CAD build for the part. Positions are in the model's coordinates, mm. A direction names the side the tool comes from. Round coordinates to 2 decimals unless told otherwise and drop trailing zeros. Write each loop counter-clockwise with the first axis right and the second up, starting at its lowest first coordinate (ties: lowest second). Pieces come first, ordered by that corner, then holes. Notation, with made-up numbers: (36, 57.25) - (73, 57.25) arc R8 cw to (73, 71.25) - close; hole circle Ø5 at (20, 67). An arc over 180 degrees is marked (long way). Put each result on its own line as item: value. Start each with the question number.
Item 1: Mould opens along X. For faces 5 (the flat face through (50.364, 6, 0)), 6 (the flat face through (16, -3, -4.645)), 7 (the cylindrical face through (55.35, 0.74, -8.24)) say: released by +X, released by -X, zero draft, split by the parting line, or undercut.
Item 2: Cut at C-C (z = -1). Give the cut face in (x, y), and give its area (3 significant figures).
Item 3: Pin check, flat tips, straight feed: pin 1 Ø3 at (x, z) = (-0.5, 4) entering from +Y; pin 2 Ø5.5 at (y, z) = (-4.5, 6.5) entering from -X; pin 3 Ø4 at (y, z) = (-3, -1.5) entering from +X. Stop position of each tip, or through.
Item 4: Cut at B-B (x = -14). Give the cut face in (y, z).
Item 5: Drill centre lines: line 1 (Y direction, x = -9.5, z = -4.5); line 2 (Y direction, x = -14, z = 6); line 3 (X direction, y = -0.5, z = -4). Where is each one in solid material? Low to high. Write a range as from..to.
Item 6: Cut at A-A (z = 18.5). Give the cut face in (x, y).
Item 7: 3-axis set-ups, long thin cutter, end or side, ignore diameter. For faces 1 (the flat face through (8.364, 6, 0)), 2 (the flat face through (51.864, -3, 7)), 3 (the flat face through (29, 6, 9.755)), 4 (the flat face through (16, -6.9, 8)): which of +Z, -Z, +X, -X, +Y, -Y reach the whole face in a straight line?
Item 8: Cut at D-D (y = -3.5). Give the cut face in (x, z).
```python
from build123d import *

# Parameters (mm, degrees)
SKETCH_1_W          = 80
SKETCH_1_H          = 36
SKETCH_1_R          = 1.5
EXTRUDE_1_DEPTH     = 1.5
SKETCH_2_W          = 71
SKETCH_2_H          = 24.2
EXTRUDE_2_DEPTH     = 7
SKETCH_3_W          = 42
SKETCH_3_H          = 19.2
EXTRUDE_3_DEPTH     = 9
SKETCH_4_W          = 64.4
SKETCH_4_H          = 14.5
CUT_EXTRUDE_1_DEPTH = 0.1


with BuildPart() as part:
    # Эскиз1 → Бобышка-Вытянуть1 (new body)
    with BuildSketch(Plane(origin=(0, 0, 0), x_dir=(1, 0, 0), z_dir=(0, 1, 0))):
        with Locations((16.363636364, -7.454545455)):
            Rectangle(SKETCH_1_W, SKETCH_1_H)
        with Locations(Location((-21.136363636, -22.954545455, 0), (0, 0, 270))):
            Circle(SKETCH_1_R, mode=Mode.SUBTRACT)
        with Locations(Location((53.863636364, 8.045454545, 0), (0, 0, 270))):
            Circle(SKETCH_1_R, mode=Mode.SUBTRACT)
        with Locations(Location((-21.136363636, 8.045454545, 0), (0, 0, 270))):
            Circle(SKETCH_1_R, mode=Mode.SUBTRACT)
        with Locations(Location((53.863636364, -22.954545455, 0), (0, 0, 270))):
            Circle(SKETCH_1_R, mode=Mode.SUBTRACT)
    extrude(amount=EXTRUDE_1_DEPTH)

    # Эскиз2 → Бобышка-Вытянуть2 (add)
    with BuildSketch(Plane.XZ):
        with Locations((16.363636364, 7.454545455)):
            Rectangle(SKETCH_2_W, SKETCH_2_H)
    extrude(amount=EXTRUDE_2_DEPTH)

    # Эскиз3 → Бобышка-Вытянуть3 (add)
    with BuildSketch(Plane(origin=(0, 1.5, 0), x_dir=(1, 0, 0), z_dir=(0, 1, 0))):
        with Locations((29.363636364, -0.154545455)):
            Rectangle(SKETCH_3_W, SKETCH_3_H)
    extrude(amount=EXTRUDE_3_DEPTH)

    # Эскиз4 → Вырез-Вытянуть1 (cut)
    with BuildSketch(Plane.XZ.offset(7)):
        with Locations((16.363636364, 7.454545455)):
            Rectangle(SKETCH_4_W, SKETCH_4_H)
    extrude(amount=-CUT_EXTRUDE_1_DEPTH, mode=Mode.SUBTRACT)


solid = part.part
```
Output values:
1. face 5: released by +X
1. face 6: zero draft
1. face 7: undercut
2. outline: (-23.64, 0) - (-19.14, 0) - (-19.14, -7) - (51.86, -7) - (51.86, 0) - (56.36, 0) - (56.36, 1.5) - (50.36, 1.5) - (50.36, 10.5) - (8.36, 10.5) - (8.36, 1.5) - (-23.64, 1.5) - close
2. area: 995 mm2
3. pin 1: y = 1.5
3. pin 2: x = -19.14
3. pin 3: x = 51.86
4. outline: (-7, -4.65) - (0, -4.65) - (0, -10.55) - (1.5, -10.55) - (1.5, 25.45) - (0, 25.45) - (0, 19.55) - (-7, 19.55) - (-7, 14.7) - (-6.9, 14.7) - (-6.9, 0.2) - (-7, 0.2) - close
5. line 1: -7..1.5
5. line 2: -6.9..1.5
5. line 3: -19.14..51.86
6. outline: (-23.64, 0) - (-19.14, 0) - (-19.14, -7) - (51.86, -7) - (51.86, 0) - (56.36, 0) - (56.36, 1.5) - (-23.64, 1.5) - close
7. face 1: +Z, -Z, -X, +Y
7. face 2: +Z, -Z, +X, -Y
7. face 3: +Z, +X, -X, +Y
7. face 4: -Y
8. outline: (-19.14, -4.65) - (51.86, -4.65) - (51.86, 19.55) - (-19.14, 19.55) - close
